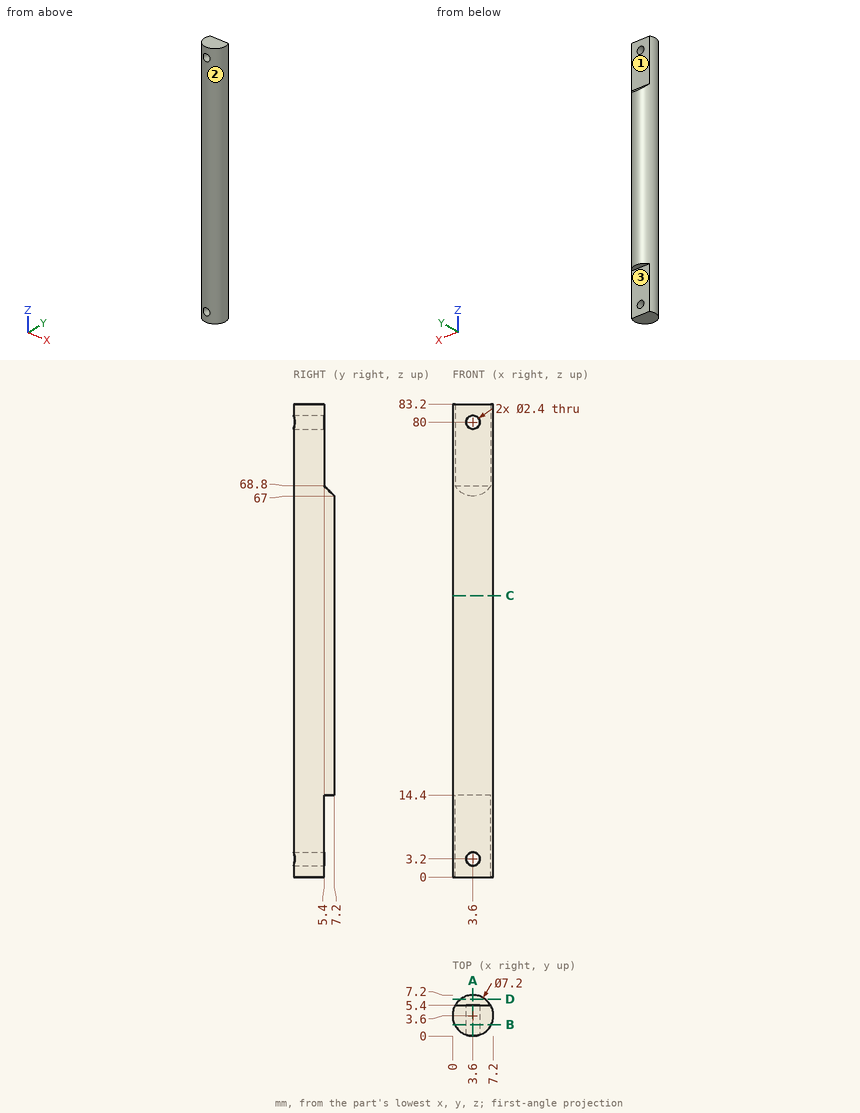
Here's the drawing with two shaded views (mm, measured from the low corner). I have some questions. A direction names the side the tool comes from. Coordinates: 2 decimals unless noted, no trailing zeros. Order: outer loops, then holes, each group sorted by start corner. A loop starts at its lowest first (then second) coordinate and runs counter-clockwise, first axis right, second up. Notation, with made-up numbers: M -24.75,44 L -5.75,44 A32 cw -5.75,73 Z; hole C 76.25,50.25 d8. An arc over 180 degrees is marked long. Write item = value, one per line.
(1) Suppose I cut it at B-B on y = 2. Please give me the cut outline in (x, z).
Results are:
outline = M 0.38,0 L 6.82,0 L 6.82,83.2 L 0.38,83.2 Z; hole C 3.6,3.2 d2.4; hole C 3.6,80 d2.4
(2) For pin 1 Ø1.5 at (y, z) = (5, 62) entering from +X; pin 2 Ø2 at (x, z) = (1.5, 53.5) entering from -Y; pin 3 Ø2 at (x, y) = (2.5, 6.5) entering from -Z, each with a flat end and sliding along its axis, tell me the tip position at first contact or that it passes through.
Results are:
pin_1 = 7.14
pin_2 = 0.17
pin_3 = 14.4
(3) For the marked faces 1, 2 and 3, which set-ups out of +Z, -Z, +X, -X, +Y, -Y let a thin tool reach every point of the face, with its end or its side?
Results are:
face_1 = +Z, +X, -X, +Y
face_2 = +Z, -Z
face_3 = -Z, +X, -X, +Y
(4) Suppose I cut it at C-C on z = 49.5. Please give me the cut outline in (x, y).
Results are:
outline = C 3.6,3.6 d7.2
(5) Suppose I cut it at A-A on x = 3.6. Please give me the cut outline in (y, z).
Results are:
outline = M 0,0 L 5.4,0 L 5.4,2 L 0,2 Z; M 0,4.4 L 5.4,4.4 L 5.4,14.4 L 7.2,14.4 L 7.2,67 L 5.4,68.8 L 5.4,78.8 L 0,78.8 Z; M 0,81.2 L 5.4,81.2 L 5.4,83.2 L 0,83.2 Z
(6) I need wall thicknesses on line 1 along Z through (x, y) = (3.75, 1.75); line 2 along Z through (x, y) = (4.5, 3); line 3 along Y through (x, z) = (3.75, 30). Which ranges of each line are inside material? Lowest first, please. Write a range as [from, to].
Results are:
line_1 = [0, 2.01], [4.39, 78.81], [81.19, 83.2]
line_2 = [0, 2.41], [3.99, 79.21], [80.79, 83.2]
line_3 = [0, 7.2]
(7) Suppose I cut it at D-D on y = 6.5. Please give me the cut outline in (x, z), plus the area to 3 significant figures.
Results are:
outline = M 1.47,14.4 L 5.73,14.4 L 5.73,67.7 L 1.47,67.7 Z
area = 227 mm2
